The drawing under review shows one solid part. Ordinate dimensions are in mm from its lowest x, y, z. A direction names the side the tool comes from. Coordinates: 2 decimals unless noted, no trailing zeros. Order: outer loops, then holes, each group sorted by start corner. A loop starts at its lowest first (then second) coordinate and runs counter-clockwise, first axis right, second up. Notation, with made-up numbers: (29, 5) -> (58, 5) arc R24 cw to (58, 39) -> close; hole circle Ø10 at (-28, 36.25). An arc over 180 degrees is marked (long way). Use a Markdown table: item, result. Add a question column.
Q1. Insertion check: pin 1 (1.5 mm diameter, centred on x = 74.5, y = 2.5, fed in from +Z); pin 2 (4 mm diameter, centred on x = 108.5, y = 11, fed in from +Z); pin 3 (3 mm diameter, centred on y = 14, z = 9, fed in from +X); pin 4 (4 mm diameter, centred on y = 11.5, z = 8.5, fed in from -X). Each pin has a flat end and moves straight along its axis. Give the tip position at first contact, or say it passes through.
Q2. Add section B-B (z = 7.5). State the section outline as (x, y) points.
Q3. Add section A-A (y = 11). State the section outline as (x, z) points (3 decimals).
Q4. Machinability: for the marked faces 1, 2 and 3, which of the approach directions +Z, -Z, +X, -X, +Y, -Y give a long, thin tool a straight path to every point of the face, cutting with its end or side? Answer none if there is none.
Q5. Wall thickness on probe 1 along Y at (x, z) = (7.5, 2.5) (3 decimals); probe 2 along X at (y, z) = (13.25, 1); probe 3 along X at (y, z) = (21.25, 6.25): over which ranges is each line inside the solid? List them lowest first.
Q6. Add section C-C (x = 108.5). State the section outline as (y, z) points (3 decimals), then the cut area to 4 significant figures.
Q7. Add section D-D (z = 1.5). State the section outline as (x, y) points (3 decimals), then the cut area to 3 significant figures.
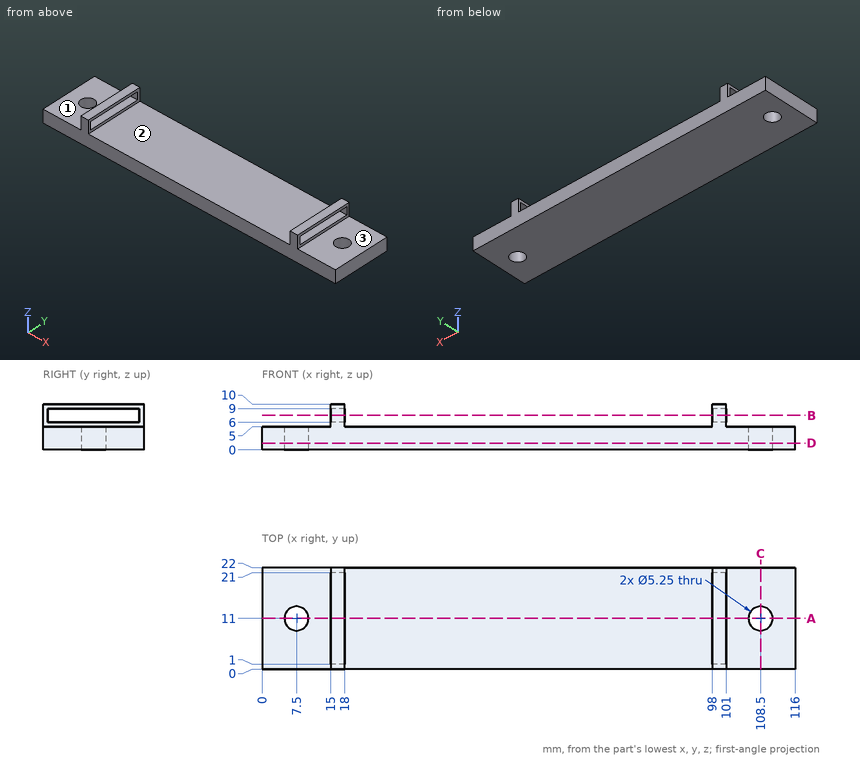
Established:
| question | item | result |
|---|---|---|
| 1 | pin 1 | z = 5 |
| 1 | pin 2 | through |
| 1 | pin 3 | x = 101 |
| 1 | pin 4 | x = 15 |
| 2 | outline | (15, 0) -> (18, 0) -> (18, 1) -> (15, 1) -> close; (15, 21) -> (18, 21) -> (18, 22) -> (15, 22) -> close; (98, 0) -> (101, 0) -> (101, 1) -> (98, 1) -> close; (98, 21) -> (101, 21) -> (101, 22) -> (98, 22) -> close |
| 3 | outline | (0, 0) -> (4.875, 0) -> (4.875, 5) -> (0, 5) -> close; (10.125, 0) -> (105.875, 0) -> (105.875, 5) -> (101, 5) -> (101, 6) -> (98, 6) -> (98, 5) -> (18, 5) -> (18, 6) -> (15, 6) -> (15, 5) -> (10.125, 5) -> close; (15, 9) -> (18, 9) -> (18, 10) -> (15, 10) -> close; (98, 9) -> (101, 9) -> (101, 10) -> (98, 10) -> close; (111.125, 0) -> (116, 0) -> (116, 5) -> (111.125, 5) -> close |
| 4 | face 1 | +Z, -X, +Y, -Y |
| 4 | face 2 | +Z, +Y, -Y |
| 4 | face 3 | +Z, +X, +Y, -Y |
| 5 | probe 1 | 0 to 8.375, 13.625 to 22 |
| 5 | probe 2 | 0 to 6.15, 8.85 to 107.15, 109.85 to 116 |
| 5 | probe 3 | 15 to 18, 98 to 101 |
| 6 | outline | (0, 0) -> (8.375, 0) -> (8.375, 5) -> (0, 5) -> close; (13.625, 0) -> (22, 0) -> (22, 5) -> (13.625, 5) -> close |
| 6 | area | 83.75 mm^2 |
| 7 | outline | (0, 0) -> (116, 0) -> (116, 22) -> (0, 22) -> close; hole circle Ø5.25 at (7.5, 11); hole circle Ø5.25 at (108.5, 11) |
| 7 | area | 2,510 mm^2 |
